Verification items for the finished model (mm, model axes). Face numbers are marked on the shaded views. A direction names the side the tool comes from. Give positions to 0.01 mm unless a question says otherwise; leave off trailing zeros. Answer as a JSON object with one key per item and string values. Group by question number.
(1) Thickness scan on line 1 (X direction, y = 19.8, z = 0); line 2 (Z direction, x = -45, y = -0.5); line 3 (Z direction, x = 0, y = 17.55). Record the ranges inside material, lowest first.
(2) Mould release check, pull along Z, two halves, no side actions. Record for the marked faces 4 and 5: +Z half, -Z half, draft (parallel to the pull), parting line (faces both ways), or undercut.
(3) Access from +Z, -Z, +X, -X, +Y, -Y to the whole of each face (thin tool, end or side, straight path). Record for the marked faces 1, 2 and 3.
(4) Depth check by flat-ended pin: pin 1 Ø21.5 at (x, z) = (-5, -3) entering from -Y; pin 2 Ø10 at (x, y) = (68.5, 10.5) entering from +Z; pin 3 Ø4 at (x, y) = (56, 9.5) entering from +Z. Enter the tip coordinate at first touch or a pass-through.
```python
from build123d import *

# Parameters (mm, degrees)
ESQUISSE1_R             = 95
BOSS_EXTRU_1_DEPTH      = 2
ESQUISSE1_12_R          = 86
ESQUISSE1_12_R_2        = 76
BOSS_EXTRU_11_DEPTH     = 4.42
ESQUISSE1_4_R           = 76
BOSS_EXTRU_3_DEPTH      = 9
ESQUISSE1_5_R           = 66
BOSS_EXTRU_4_DEPTH      = 12.8
ESQUISSE1_6_R           = 56
BOSS_EXTRU_5_DEPTH      = 16
ESQUISSE1_7_R           = 46
BOSS_EXTRU_6_DEPTH      = 18.8
ESQUISSE1_8_R           = 36
BOSS_EXTRU_7_DEPTH      = 21
ESQUISSE1_9_R           = 26
BOSS_EXTRU_8_DEPTH      = 22.5
ESQUISSE1_10_R          = 16
BOSS_EXTRU_9_DEPTH      = 23.7
COQUE1_START            = -2
COQUE1_OUTLINE_R        = 64
COQUE1_DEPTH            = 12.8
COQUE1_2_OUTLINE_R      = 84
COQUE1_2_OUTLINE_R_2    = 64
COQUE1_2_DEPTH          = 4.42
COQUE1_START_2          = 10.8
COQUE1_3_OUTLINE_R      = 44
COQUE1_3_DEPTH          = 6
COQUE1_START_3          = 2.42
COQUE1_4_OUTLINE_R      = 74
COQUE1_4_OUTLINE_R_2    = 64
COQUE1_4_DEPTH          = 4.58
COQUE1_5_OUTLINE_R      = 54
COQUE1_5_OUTLINE_R_2    = 44
COQUE1_5_DEPTH          = 3.2
COQUE1_START_4          = 16.8
COQUE1_6_OUTLINE_R      = 34
COQUE1_6_DEPTH          = 2.2
COQUE1_START_5          = 19
COQUE1_7_OUTLINE_R      = 24
COQUE1_7_DEPTH          = 1.5
COQUE1_START_6          = 20.5
COQUE1_8_OUTLINE_R      = 14
COQUE1_8_DEPTH          = 1.2
ESQUISSE4_W             = 5
ESQUISSE4_H             = 12
ENL_V_MAT_EXTRU_2_DEPTH = 137.786293173
D_GAGEMENT_M31_D        = 3.4


# Read off the part's stored shape, not the designer's step: Coque1
with BuildPart() as part:
    # Esquisse1 → Boss.-Extru.1 (new body)
    with BuildSketch(Plane(origin=(0, 0, 0), x_dir=(1, 0, 0), z_dir=(0, 1, 0))):
        with Locations(Location((0, 0, 0), (0, 0, 270))):
            Circle(ESQUISSE1_R)
    extrude(amount=-BOSS_EXTRU_1_DEPTH)

    # Esquisse1<12> → Boss.-Extru.11 (add)
    with BuildSketch(Plane(origin=(0, 0, 0), x_dir=(1, 0, 0), z_dir=(0, 1, 0))):
        with Locations(Location((0, 0, 0), (0, 0, 270))):
            Circle(ESQUISSE1_12_R)
        with Locations(Location((0, 0, 0), (0, 0, 270))):
            Circle(ESQUISSE1_12_R_2, mode=Mode.SUBTRACT)
    extrude(amount=BOSS_EXTRU_11_DEPTH)

    # Esquisse1<4> → Boss.-Extru.3 (add)
    with BuildSketch(Plane(origin=(0, 0, 0), x_dir=(1, 0, 0), z_dir=(0, 1, 0))):
        with Locations(Location((0, 0, 0), (0, 0, 270))):
            Circle(ESQUISSE1_4_R)
    extrude(amount=BOSS_EXTRU_3_DEPTH)

    # Esquisse1<5> → Boss.-Extru.4 (add)
    with BuildSketch(Plane(origin=(0, 0, 0), x_dir=(1, 0, 0), z_dir=(0, 1, 0))):
        with Locations(Location((0, 0, 0), (0, 0, 270))):
            Circle(ESQUISSE1_5_R)
    extrude(amount=BOSS_EXTRU_4_DEPTH)

    # Esquisse1<6> → Boss.-Extru.5 (add)
    with BuildSketch(Plane(origin=(0, 0, 0), x_dir=(1, 0, 0), z_dir=(0, 1, 0))):
        with Locations(Location((0, 0, 0), (0, 0, 270))):
            Circle(ESQUISSE1_6_R)
    extrude(amount=BOSS_EXTRU_5_DEPTH)

    # Esquisse1<7> → Boss.-Extru.6 (add)
    with BuildSketch(Plane(origin=(0, 0, 0), x_dir=(1, 0, 0), z_dir=(0, 1, 0))):
        with Locations(Location((0, 0, 0), (0, 0, 270))):
            Circle(ESQUISSE1_7_R)
    extrude(amount=BOSS_EXTRU_6_DEPTH)

    # Esquisse1<8> → Boss.-Extru.7 (add)
    with BuildSketch(Plane(origin=(0, 0, 0), x_dir=(1, 0, 0), z_dir=(0, 1, 0))):
        with Locations(Location((0, 0, 0), (0, 0, 90))):
            Circle(ESQUISSE1_8_R)
    extrude(amount=BOSS_EXTRU_7_DEPTH)

    # Esquisse1<9> → Boss.-Extru.8 (add)
    with BuildSketch(Plane(origin=(0, 0, 0), x_dir=(1, 0, 0), z_dir=(0, 1, 0))):
        with Locations(Location((0, 0, 0), (0, 0, 270))):
            Circle(ESQUISSE1_9_R)
    extrude(amount=BOSS_EXTRU_8_DEPTH)

    # Esquisse1<10> → Boss.-Extru.9 (add)
    with BuildSketch(Plane(origin=(0, 0, 0), x_dir=(1, 0, 0), z_dir=(0, 1, 0))):
        with Locations(Location((0, 0, 0), (0, 0, 270))):
            Circle(ESQUISSE1_10_R)
    extrude(amount=BOSS_EXTRU_9_DEPTH)

    # Coque1 outline → Coque1 (cut)
    with BuildSketch(Plane(origin=(0, 0, 0), x_dir=(1, 0, 0), z_dir=(0, 1, 0)).offset(COQUE1_START)):
        Circle(COQUE1_OUTLINE_R)
    extrude(amount=COQUE1_DEPTH, mode=Mode.SUBTRACT)

    # Coque1 2 outline → Coque1 2 (cut)
    with BuildSketch(Plane(origin=(0, 0, 0), x_dir=(1, 0, 0), z_dir=(0, 1, 0)).offset(COQUE1_START)):
        Circle(COQUE1_2_OUTLINE_R)
        Circle(COQUE1_2_OUTLINE_R_2, mode=Mode.SUBTRACT)
    extrude(amount=COQUE1_2_DEPTH, mode=Mode.SUBTRACT)

    # Coque1 3 outline → Coque1 3 (cut)
    with BuildSketch(Plane(origin=(0, 0, 0), x_dir=(1, 0, 0), z_dir=(0, 1, 0)).offset(COQUE1_START_2)):
        Circle(COQUE1_3_OUTLINE_R)
    extrude(amount=COQUE1_3_DEPTH, mode=Mode.SUBTRACT)

    # Coque1 4 outline → Coque1 4 (cut)
    with BuildSketch(Plane(origin=(0, 0, 0), x_dir=(1, 0, 0), z_dir=(0, 1, 0)).offset(COQUE1_START_3)):
        Circle(COQUE1_4_OUTLINE_R)
        Circle(COQUE1_4_OUTLINE_R_2, mode=Mode.SUBTRACT)
    extrude(amount=COQUE1_4_DEPTH, mode=Mode.SUBTRACT)

    # Coque1 5 outline → Coque1 5 (cut)
    with BuildSketch(Plane(origin=(0, 0, 0), x_dir=(1, 0, 0), z_dir=(0, 1, 0)).offset(COQUE1_START_2)):
        Circle(COQUE1_5_OUTLINE_R)
        Circle(COQUE1_5_OUTLINE_R_2, mode=Mode.SUBTRACT)
    extrude(amount=COQUE1_5_DEPTH, mode=Mode.SUBTRACT)

    # Coque1 6 outline → Coque1 6 (cut)
    with BuildSketch(Plane(origin=(0, 0, 0), x_dir=(1, 0, 0), z_dir=(0, 1, 0)).offset(COQUE1_START_4)):
        Circle(COQUE1_6_OUTLINE_R)
    extrude(amount=COQUE1_6_DEPTH, mode=Mode.SUBTRACT)

    # Coque1 7 outline → Coque1 7 (cut)
    with BuildSketch(Plane(origin=(0, 0, 0), x_dir=(1, 0, 0), z_dir=(0, 1, 0)).offset(COQUE1_START_5)):
        Circle(COQUE1_7_OUTLINE_R)
    extrude(amount=COQUE1_7_DEPTH, mode=Mode.SUBTRACT)

    # Coque1 8 outline → Coque1 8 (cut)
    with BuildSketch(Plane(origin=(0, 0, 0), x_dir=(1, 0, 0), z_dir=(0, 1, 0)).offset(COQUE1_START_6)):
        Circle(COQUE1_8_OUTLINE_R)
    extrude(amount=COQUE1_8_DEPTH, mode=Mode.SUBTRACT)

    # Esquisse4 → Enlèv. mat.-Extru.2 (cut, through all)
    with BuildSketch(Plane(origin=(0, 23.7, 0), x_dir=(1, 0, 0), z_dir=(0, 1, 0))):
        with Locations((-21.5, 0)):
            Rectangle(ESQUISSE4_W, ESQUISSE4_H)
        Rectangle(ESQUISSE4_W, ESQUISSE4_H)
        with Locations((-11.5, 0)):
            Rectangle(ESQUISSE4_W, ESQUISSE4_H)
        with Locations((-31.5, 0)):
            Rectangle(ESQUISSE4_W, ESQUISSE4_H)
        with Locations((-41.5, 0)):
            Rectangle(ESQUISSE4_W, ESQUISSE4_H)
        with Locations((-51.5, 0)):
            Rectangle(ESQUISSE4_W, ESQUISSE4_H)
        with Locations((-61.5, 0)):
            Rectangle(ESQUISSE4_W, ESQUISSE4_H)
        with Locations((-71.5, 0)):
            Rectangle(ESQUISSE4_W, ESQUISSE4_H)
        with Locations((-81.5, 0)):
            Rectangle(ESQUISSE4_W, ESQUISSE4_H)
    extrude(amount=-ENL_V_MAT_EXTRU_2_DEPTH, mode=Mode.SUBTRACT)

    # Dégagement M31 (through all)
    with Locations(Plane(origin=(0, 0, 0), x_dir=(1, 0, 0), z_dir=(0, 1, 0))):
        with Locations((90, 0), (-45, 77.942286341), (-45, -77.942286341)):
            Hole(D_GAGEMENT_M31_D / 2)


solid = part.part
```
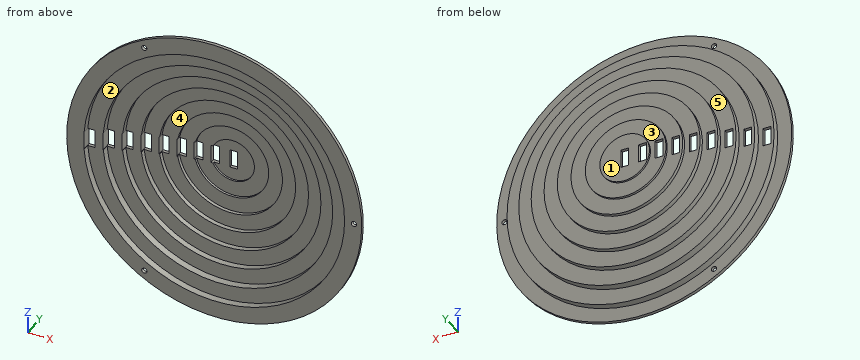
Solutions:
{
 "1": {"line 1": "x = -36 to -34, -29 to -24, 24 to 36", "line 2": "z = -83.67 to -79.64, -76.24 to -70.93, 70.93 to 76.24, 79.64 to 83.67", "line 3": "z = -46 to -34, 34 to 46"},
 "2": {"face 4": "undercut", "face 5": "draft"},
 "3": {"face 1": "+Z, -Z, +X, -X, +Y", "face 2": "-Y", "face 3": "+Y"},
 "4": {"pin 1": "stops at y = 20.5", "pin 2": "stops at z = 41.41", "pin 3": "stops at z = 53.41"}
}
